Design review of the part built by this model. Coordinates are the model's own, in mm. Face numbers are marked on the shaded views. Give positions to 0.01 mm unless a question says otherwise; leave off trailing zeros. Order: outer loops, then holes, each group sorted by start corner. A loop starts at its lowest first (then second) coordinate and runs counter-clockwise, first axis right, second up. Notation, with made-up numbers: (86, 38) -> (99, 38) arc R20 ccw to (99, 59) -> close; hole circle Ø10 at (67.5, 34). An arc over 180 degrees is marked (long way). Use a Markdown table: item, result. Add a question column.
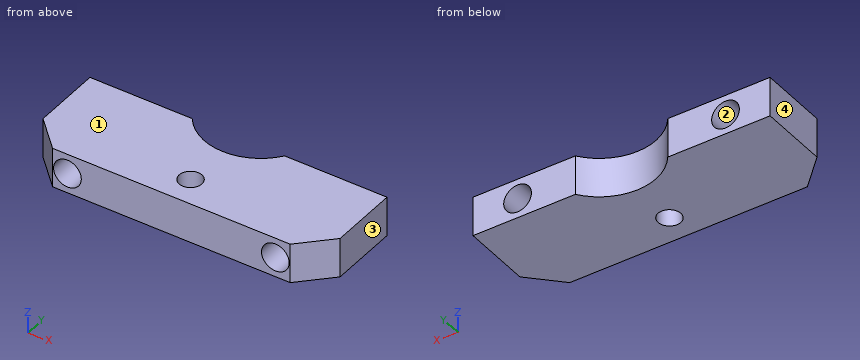
```python
from build123d import *

# Parameters (mm, degrees)
SKETCH_1_W          = 30
SKETCH_1_H          = 13
EXTRUDE_1_DEPTH     = 4
SKETCH_3_R          = 5.75
CUT_EXTRUDE_2_DEPTH = 10
SKETCH_7_W          = 30
SKETCH_7_H          = 3
CUT_EXTRUDE_3_DEPTH = 10
CHAMFER_1_SIZE      = 3
SKETCH_8_R          = 1.4
CUT_EXTRUDE_4_DEPTH = 19.466185313
SKETCH_5_R          = 1.15
CUT_EXTRUDE_5_DEPTH = 10


with BuildPart() as part:
    # 草图1 → 凸台-拉伸1 (new body)
    with BuildSketch(Plane.XY):
        Rectangle(SKETCH_1_W, SKETCH_1_H)
    extrude(amount=EXTRUDE_1_DEPTH)

    # 草图3 → 切除-拉伸2 (cut)
    with BuildSketch(Plane.XY.offset(4)):
        with Locations((0, 9.854101966)):
            Circle(SKETCH_3_R)
    extrude(amount=-CUT_EXTRUDE_2_DEPTH, mode=Mode.SUBTRACT)

    # 草图7 → 切除-拉伸3 (cut)
    with BuildSketch(Plane.XY.offset(4)):
        with Locations((0, -5)):
            Rectangle(SKETCH_7_W, SKETCH_7_H)
    extrude(amount=-CUT_EXTRUDE_3_DEPTH, mode=Mode.SUBTRACT)

    # 倒角1
    chamfer_1_edges = [part.edges().sort_by_distance(p)[0] for p in [
        (-15, -3.5, 2),
        (15, -3.5, 2),
    ]]
    chamfer(chamfer_1_edges, length=CHAMFER_1_SIZE)

    # 草图8 → 切除-拉伸4 (cut, through all)
    with BuildSketch(Plane.XZ.offset(3.5)):
        with Locations(Location((-10.5, 2, 0), (0, 0, 270))):
            Circle(SKETCH_8_R)
    cut_extrude_4 = extrude(amount=-CUT_EXTRUDE_4_DEPTH, mode=Mode.SUBTRACT)

    # 镜向1: 切除-拉伸4 across plane
    add(cut_extrude_4.mirror(Plane(origin=(0, 0, 0), x_dir=(0, 0, 1), z_dir=(1, 0, 0))), mode=Mode.SUBTRACT)

    # 草图5 → 切除-拉伸5 (cut)
    with BuildSketch(Plane.XY.offset(4)):
        with Locations((0, -0.645898034)):
            Circle(SKETCH_5_R)
    extrude(amount=-CUT_EXTRUDE_5_DEPTH, mode=Mode.SUBTRACT)


solid = part.part
```
1) The part is to be moulded in two halves that separate along X. For the marked faces 1, 2, 3 and 4, say which applies: +X half, -X half, draft (parallel to the pull), parting line (faces both ways), or undercut.
2) Add section A-A (x = 0). Give the boundary of the cut face in (y, z).
3) Add section D-D (x = 10.5). Give the boundary of the cut face in (y, z).
4) For L1, parallel to X at y = 3.5, z = 2; L2, parallel to Y at x = 0, z = 2.4; L3, parallel to Z at x = 10.5, y = 1.25, list the stretches that pass through material, from the lowest coordinate up. Write a range as [from, to].
5) Add section B-B (z = 2.1). Give the boundary of the cut face in (x, y).
6) Add section C-C (y = 5). Give the boundary of the cut face in (x, z), then the cut area to 3 significant figures.
7) Insertion check: pin 1 (1.7 mm diameter, centred on x = -10.5, z = 2, fed in from +Y). The pin has a flat end and moves straight along its axis. Give the tip position at first contact, or say it passes through.
Worked answers:
| question | item | result |
|---|---|---|
| 1 | face 1 | draft |
| 1 | face 2 | undercut |
| 1 | face 3 | +X half |
| 1 | face 4 | -X half |
| 2 | outline | (-3.5, 0) -> (-1.8, 0) -> (-1.8, 4) -> (-3.5, 4) -> close; (0.5, 0) -> (4.1, 0) -> (4.1, 4) -> (0.5, 4) -> close |
| 3 | outline | (-3.5, 0) -> (6.5, 0) -> (6.5, 0.6) -> (-3.5, 0.6) -> close; (-3.5, 3.4) -> (6.5, 3.4) -> (6.5, 4) -> (-3.5, 4) -> close |
| 4 | L1 | [-15, -11.9], [-9.1, 9.1], [11.9, 15] |
| 4 | L2 | [-3.5, -1.8], [0.5, 4.1] |
| 4 | L3 | [0, 0.6], [3.4, 4] |
| 5 | outline | (-15, -0.5) -> (-12, -3.5) -> (-11.9, -3.5) -> (-11.9, 6.5) -> (-15, 6.5) -> close; (-9.1, -3.5) -> (9.1, -3.5) -> (9.1, 6.5) -> (4.67, 6.5) arc R5.75 cw to (-4.67, 6.5) -> (-9.1, 6.5) -> close; (11.9, -3.5) -> (12, -3.5) -> (15, -0.5) -> (15, 6.5) -> (11.9, 6.5) -> close; hole circle Ø2.3 at (0, -0.65) |
| 6 | outline | (-15, 0) -> (-3.08, 0) -> (-3.08, 4) -> (-15, 4) -> close; (3.08, 0) -> (15, 0) -> (15, 4) -> (3.08, 4) -> close; hole circle Ø2.8 at (-10.5, 2); hole circle Ø2.8 at (10.5, 2) |
| 6 | area | 83.0 mm^2 |
| 7 | pin 1 | through |
